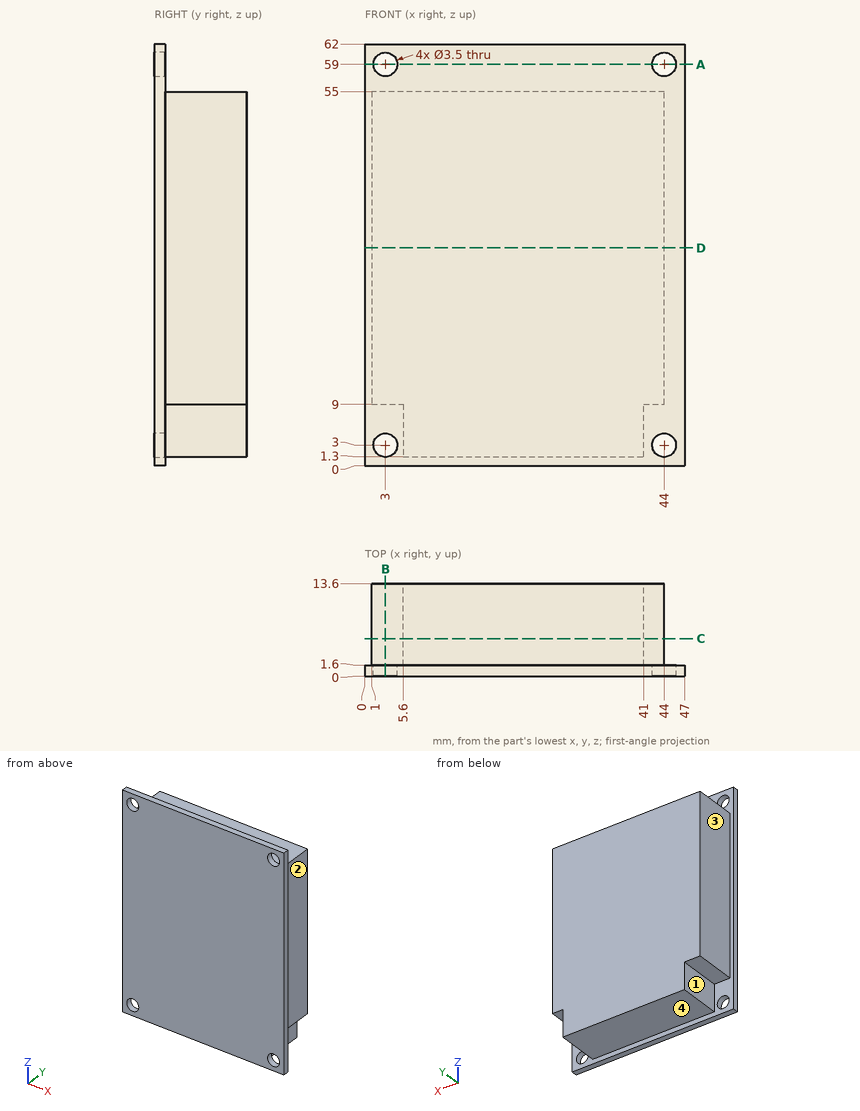
The drawing under review shows one solid part. Ordinate dimensions are in mm from its lowest x, y, z. A direction names the side the tool comes from. Coordinates: 2 decimals unless noted, no trailing zeros. Order: outer loops, then holes, each group sorted by start corner. A loop starts at its lowest first (then second) coordinate and runs counter-clockwise, first axis right, second up. Notation, with made-up numbers: (-40, 22) -> (-6, 22) arc R23 ccw to (-6, 56) -> close; hole circle Ø1 at (58, 19.25). An arc over 180 degrees is marked (long way). Answer in a Markdown table with one row per item. Add a question column.
Item 1: Clearance check with flat-ended pins moving along their axes: pin 1 (2 mm diameter, centred on x = 44, z = 59, fed in from +Y); pin 2 (2.5 mm diameter, centred on x = 42.5, y = 6, fed in from -Z); pin 3 (5 mm diameter, centred on y = 11.5, z = 33, fed in from -X); pin 4 (6 mm diameter, centred on y = 10.5, z = 17.5, fed in from +X). State where each tip first meets the part, or that it passes through.
Item 2: We need section C-C on y = 5.5. Write out the cut boundary in (x, z), plus the area to 3 significant figures.
Item 3: We need section A-A on z = 59. Write out the cut boundary in (x, y).
Item 4: Machinability: for the marked faces 1, 2, 3 and 4, which of the approach directions +Z, -Z, +X, -X, +Y, -Y give a long, thin tool a straight path to every point of the face, cutting with its end or side? Answer none if there is none.
Item 5: We need section D-D on z = 32. Write out the cut boundary in (x, y), plus the area to 3 significant figures.
Item 6: To check wall thickness, follow probe 1 along X at (y, z) = (1.05, 3); probe 2 along X at (y, z) = (3.5, 48.5); probe 3 along X at (y, z) = (2.5, 5). State the ranges of each line that lie inside material, in increasing order.
Item 7: We need section B-B on x = 3. Write out the cut boundary in (y, z).
Final values:
| question | item | result |
|---|---|---|
| 1 | pin 1 | passes through |
| 1 | pin 2 | stops at z = 9 |
| 1 | pin 3 | stops at x = 1 |
| 1 | pin 4 | stops at x = 44 |
| 2 | outline | (1, 9) -> (5.6, 9) -> (5.6, 1.3) -> (41, 1.3) -> (41, 9) -> (44, 9) -> (44, 55) -> (1, 55) -> close |
| 2 | area | 2,250 mm2 |
| 3 | outline | (0, 0) -> (1.25, 0) -> (1.25, 1.6) -> (0, 1.6) -> close; (4.75, 0) -> (42.25, 0) -> (42.25, 1.6) -> (4.75, 1.6) -> close; (45.75, 0) -> (47, 0) -> (47, 1.6) -> (45.75, 1.6) -> close |
| 4 | face 1 | -Z, -X, +Y |
| 4 | face 2 | +Z, -Z, +X, +Y |
| 4 | face 3 | +Z, -Z, -X, +Y |
| 4 | face 4 | -Z, +X, -X, +Y |
| 5 | outline | (0, 0) -> (47, 0) -> (47, 1.6) -> (44, 1.6) -> (44, 13.6) -> (1, 13.6) -> (1, 1.6) -> (0, 1.6) -> close |
| 5 | area | 591 mm2 |
| 6 | probe 1 | x = 0 to 1.25, 4.75 to 42.25, 45.75 to 47 |
| 6 | probe 2 | x = 1 to 44 |
| 6 | probe 3 | x = 5.6 to 41 |
| 7 | outline | (0, 0) -> (1.6, 0) -> (1.6, 1.25) -> (0, 1.25) -> close; (0, 4.75) -> (1.6, 4.75) -> (1.6, 9) -> (13.6, 9) -> (13.6, 55) -> (1.6, 55) -> (1.6, 57.25) -> (0, 57.25) -> close; (0, 60.75) -> (1.6, 60.75) -> (1.6, 62) -> (0, 62) -> close |
